Part model, mm, in its own coordinate system. A direction names the side the tool comes from. Round coordinates to 2 decimals unless told otherwise and drop trailing zeros. Write each question's results on one line, items separated by ' | '.
from build123d import *

# Parameters (mm, degrees)
F0_R     = 3.1
F0_R_2   = 22.5
F1_DEPTH = 6
F2_SIZE2 = 3
F2_SIZE  = 3
F3_SIZE2 = 5
F3_SIZE  = 5
F4_SIZE  = 5
F5_SIZE2 = 5
F5_SIZE  = 5


with BuildPart() as f1:
    # F0 (on Front) → F1 (new body)
    with BuildSketch(Plane.XZ):
        with BuildLine():
            ThreePointArc((-10.045547, 56.971129), (-37.185263, -44.315671), (57.85, 0))
            ThreePointArc((57.85, 0), (37.185263, 44.315671), (-10.045547, 56.971129))
        make_face()
        with Locations((-21.5, -37.239092)):
            Circle(F0_R, mode=Mode.SUBTRACT)
        with BuildLine():
            ThreePointArc((-23.382686, 13.5), (-24.368717, 11.626075), (-25.204864, 9.680642))
            ThreePointArc((-25.204864, 9.680642), (-27, 0), (-25.204864, -9.680642))
            ThreePointArc((-25.204864, -9.680642), (-24.368717, -11.626075), (-23.382686, -13.5))
            ThreePointArc((-23.382686, -13.5), (-23.262708, -13.705708), (-23.14092, -13.91035))
            ThreePointArc((-23.14092, -13.91035), (-22.49477, -17.311118), (-24.212337, -20.316563))
            Line((-24.212337, -20.316563), (-34.258549, -28.746336))
            ThreePointArc((-34.258549, -28.746336), (-38.184741, -29.865123), (-41.636097, -27.684571))
            ThreePointArc((-41.636097, -27.684571), (-42.489891, -26.35544), (-43.30127, -25))
            ThreePointArc((-43.30127, -25), (-44.625232, -22.551911), (-45.810926, -20.033948))
            ThreePointArc((-45.810926, -20.033948), (-50, 0), (-45.810926, 20.033948))
            ThreePointArc((-45.810926, 20.033948), (-44.625232, 22.551911), (-43.30127, 25))
            ThreePointArc((-43.30127, 25), (-42.489891, 26.35544), (-41.636097, 27.684571))
            ThreePointArc((-41.636097, 27.684571), (-38.184741, 29.865123), (-34.258549, 28.746336))
            Line((-34.258549, 28.746336), (-24.212337, 20.316563))
            ThreePointArc((-24.212337, 20.316563), (-22.49477, 17.311118), (-23.14092, 13.91035))
            ThreePointArc((-23.14092, 13.91035), (-23.262708, 13.705708), (-23.382686, 13.5))
        make_face(mode=Mode.SUBTRACT)
        Circle(F0_R_2, mode=Mode.SUBTRACT)
        with BuildLine():
            ThreePointArc((4.21875, -26.668374), (13.5, -23.382686), (20.986114, -16.987731))
            ThreePointArc((20.986114, -16.987731), (22.252835, -15.29089), (23.382686, -13.5))
            ThreePointArc((23.382686, -13.5), (23.500845, -13.293242), (23.617176, -13.085449))
            ThreePointArc((23.617176, -13.085449), (26.239253, -10.825483), (29.700828, -10.810217))
            Line((29.700828, -10.810217), (42.024332, -15.295606))
            ThreePointArc((42.024332, -15.295606), (44.956326, -18.136394), (44.79359, -22.215632))
            ThreePointArc((44.79359, -22.215632), (44.069426, -23.619605), (43.30127, -25))
            ThreePointArc((43.30127, -25), (41.843144, -27.370629), (40.255371, -29.656452))
            ThreePointArc((40.255371, -29.656452), (25, -43.30127), (5.555556, -49.690399))
            ThreePointArc((5.555556, -49.690399), (2.782088, -49.92254), (0, -50))
            ThreePointArc((0, -50), (-1.579535, -49.975044), (-3.157493, -49.900203))
            ThreePointArc((-3.157493, -49.900203), (-6.771585, -48.001517), (-7.765783, -44.041942))
            Line((-7.765783, -44.041942), (-5.488491, -31.12678))
            ThreePointArc((-5.488491, -31.12678), (-3.744483, -28.136601), (-0.476257, -26.995799))
            ThreePointArc((-0.476257, -26.995799), (-0.238138, -26.99895), (0, -27))
            ThreePointArc((0, -27), (2.115882, -26.916966), (4.21875, -26.668374))
        make_face(mode=Mode.SUBTRACT)
        with BuildLine():
            ThreePointArc((39.9, 0), (43, 3.1), (46.1, 0))
            ThreePointArc((46.1, 0), (43, -3.1), (39.9, 0))
        make_face(mode=Mode.SUBTRACT)
        with Locations((-21.5, 37.239092)):
            Circle(F0_R, mode=Mode.SUBTRACT)
        with BuildLine():
            ThreePointArc((20.986114, 16.987731), (13.5, 23.382686), (4.21875, 26.668374))
            ThreePointArc((4.21875, 26.668374), (1.878394, 26.934581), (-0.476257, 26.995799))
            ThreePointArc((-0.476257, 26.995799), (-3.744483, 28.136601), (-5.488491, 31.12678))
            Line((-5.488491, 31.12678), (-7.765783, 44.041942))
            ThreePointArc((-7.765783, 44.041942), (-6.771585, 48.001517), (-3.157493, 49.900203))
            ThreePointArc((-3.157493, 49.900203), (1.203611, 49.985511), (5.555556, 49.690399))
            ThreePointArc((5.555556, 49.690399), (25, 43.30127), (40.255371, 29.656452))
            ThreePointArc((40.255371, 29.656452), (42.686917, 26.035114), (44.79359, 22.215632))
            ThreePointArc((44.79359, 22.215632), (44.956326, 18.136394), (42.024332, 15.295606))
            Line((42.024332, 15.295606), (29.700828, 10.810217))
            ThreePointArc((29.700828, 10.810217), (26.239253, 10.825483), (23.617176, 13.085449))
            ThreePointArc((23.617176, 13.085449), (22.386834, 15.094028), (20.986114, 16.987731))
        make_face(mode=Mode.SUBTRACT)
    extrude(amount=F1_DEPTH)

    # F2
    f2_edges = [f1.edges().sort_by_distance(p)[0] for p in [
        (-22.5, -6, 0),
    ]]
    chamfer(f2_edges, length=F2_SIZE, length2=F2_SIZE2)

    # F3
    f3_edges = [f1.edges().sort_by_distance(p)[0] for p in [
        (-24.6, -6, 37.239092),
    ]]
    chamfer(f3_edges, length=F3_SIZE, length2=F3_SIZE2)

    # F4
    f4_edges = [f1.edges().sort_by_distance(p)[0] for p in [
        (-24.6, -6, -37.239092),
    ]]
    chamfer(f4_edges, length=F4_SIZE)

    # F5
    f5_edges = [f1.edges().sort_by_distance(p)[0] for p in [
        (39.9, -6, 0),
    ]]
    chamfer(f5_edges, length=F5_SIZE, length2=F5_SIZE2)


solid = f1.part
Item 1: Band-saw the part on A-A on y = -5.05. Count the separate pieces of the cut face and the enclosed holes in it, and give its area (3 significant figures).
Filled sheet:
separate pieces: 1 | enclosed holes: 7 | area: 4,490 mm^2
Item 2: Wall check: L1, parallel to X at y = -1.95, z = 40; L2, parallel to X at y = -3.25, z = 19; L3, parallel to X at y = -2.5, z = -41. Give the ranges that are in metal, low to high.
Filled sheet:
L1: -41.79 to -24.46, -18.54 to -7.05, 30 to 41.79 | L2: -54.64 to -46.25, -23.1 to -12.51, 12.51 to 19.18, 45.21 to 54.64 | L3: -40.81 to -24.15, -18.85 to -7.23, 28.62 to 40.81
Item 3: Two-plate mould, pull along Z, no slides. Class faces 1 (the conical face through (-21.94, -1.24, 40.55)), 2 (the flat face through (-1, 0, -25)): +Z half, -Z half, draft (parallel to the pull), parting line (faces both ways), or undercut.
Filled sheet:
face 1: undercut | face 2: draft
Item 4: Which spindle directions (+Z, -Z, +X, -X, +Y, -Y) get a long thin tool onto all of the face, cutting with end or side? Do faces 3 (the cylindrical face through (13.62, -2.958, 23.313)), 4 (the conical face through (21.64, -3.188, 6.815)). Say none if no direction does.
Filled sheet:
face 3: +Y, -Y | face 4: -Y
Item 5: Drop flat-ended pins along their axis: P1, Ø10, axis at x = 43, z = 0, coming from the -Y side; P2, Ø6, axis at x = 37.5, z = 3.5, coming from the +Y side; P3, Ø3, axis at x = -39.5, y = -4.5, coming from the +Z side; P4, Ø2, axis at x = 6, y = -1, coming from the +Z side. Give the stop position or say it passes through.
Filled sheet:
P1: y = -2.9 | P2: y = 0 | P3: z = 43.62 | P4: z = 57.63
